Verification items for the finished model (mm, model axes). Give positions to 0.01 mm unless a question says otherwise; leave off trailing zeros. Order: outer loops, then holes, each group sorted by start corner. A loop starts at its lowest first (then second) coordinate and runs counter-clockwise, first axis right, second up.
from build123d import *
from OCP.BRepFilletAPI import BRepFilletAPI_MakeChamfer

# Parameters (mm, degrees)
SKETCH1_W           = 3.53
SKETCH1_H           = 9.2
BOSS_EXTRUDE1_DEPTH = 4
BOSS_EXTRUDE2_DEPTH = 4
CHAMFER1_SIZE       = 1.5
CHAMFER1_SIZE2      = 0.5
CHAMFER2_SIZE       = 0.5
CHAMFER2_SIZE2      = 1.5


with BuildPart() as part:
    # Sketch1 → Boss-Extrude1 (new body)
    with BuildSketch(Plane.XY):
        Polygon((52.4925, 30), (52.4925, -30), (-54.2075, -30), (-54.2075, 14), (-68.2075, 14), (-68.2075, 30), align=None)
        with BuildLine():
            Line((-31.510630119, 17.647843267), (22.89855475, 17.647843267))
            ThreePointArc((22.89855475, 17.647843267), (-4.306037684, -22.627990687), (-31.510630119, 17.647843267))
        make_face(mode=Mode.SUBTRACT)
        with Locations((-39.0075, 21.35)):
            Rectangle(SKETCH1_W, SKETCH1_H, mode=Mode.SUBTRACT)
        with Locations((45.7925, 20.65)):
            Rectangle(SKETCH1_W, SKETCH1_H, mode=Mode.SUBTRACT)
        with Locations((45.8, -20.65)):
            Rectangle(SKETCH1_W, SKETCH1_H, mode=Mode.SUBTRACT)
        with Locations((-64.9075, 21.35)):
            Rectangle(SKETCH1_W, SKETCH1_H, mode=Mode.SUBTRACT)
    extrude(amount=BOSS_EXTRUDE1_DEPTH)

    # Sketch2 → Boss-Extrude2 (add)
    with BuildSketch(Plane.XY):
        Polygon((-68.2075, 30), (52.4925, 30), (52.4925, 55), (37.4925, 55), (23.350364376, 40.857864376), (-39.065364376, 40.857864376), (-53.2075, 55), (-68.2075, 55), align=None)
    extrude(amount=BOSS_EXTRUDE2_DEPTH)

    # Chamfer1: one chamfer whose edges measure the first distance from different faces: ONE call of the kernel's chamfer builder (chamfer() names one face for all edges)
    chamfer1_edges_1 = [part.edges().sort_by_distance(p)[0] for p in [
        (-40.7725, 21.35, 0),
    ]]
    chamfer1_side_1 = [part.faces().sort_by_distance(p)[0] for p in [
        (-40.7725, 21.35, 2),
    ]]
    chamfer1_edges_2 = [part.edges().sort_by_distance(p)[0] for p in [
        (-39.0075, 16.75, 0),
    ]]
    chamfer1_side_2 = [part.faces().sort_by_distance(p)[0] for p in [
        (-39.0075, 16.75, 2),
    ]]
    chamfer1_edges_3 = [part.edges().sort_by_distance(p)[0] for p in [
        (-37.2425, 21.35, 0),
    ]]
    chamfer1_side_3 = [part.faces().sort_by_distance(p)[0] for p in [
        (-37.2425, 21.35, 2),
    ]]
    chamfer1_edges_4 = [part.edges().sort_by_distance(p)[0] for p in [
        (-39.0075, 25.95, 0),
    ]]
    chamfer1_side_4 = [part.faces().sort_by_distance(p)[0] for p in [
        (-39.0075, 25.95, 2),
    ]]
    chamfer1_edges_5 = [part.edges().sort_by_distance(p)[0] for p in [
        (-66.6725, 21.35, 0),
    ]]
    chamfer1_side_5 = [part.faces().sort_by_distance(p)[0] for p in [
        (-66.6725, 21.35, 2),
    ]]
    chamfer1_edges_6 = [part.edges().sort_by_distance(p)[0] for p in [
        (-64.9075, 16.75, 0),
    ]]
    chamfer1_side_6 = [part.faces().sort_by_distance(p)[0] for p in [
        (-64.9075, 16.75, 2),
    ]]
    chamfer1_edges_7 = [part.edges().sort_by_distance(p)[0] for p in [
        (-63.1425, 21.35, 0),
    ]]
    chamfer1_side_7 = [part.faces().sort_by_distance(p)[0] for p in [
        (-63.1425, 21.35, 2),
    ]]
    chamfer1_edges_8 = [part.edges().sort_by_distance(p)[0] for p in [
        (-64.9075, 25.95, 0),
    ]]
    chamfer1_side_8 = [part.faces().sort_by_distance(p)[0] for p in [
        (-64.9075, 25.95, 2),
    ]]
    chamfer1_edges_9 = [part.edges().sort_by_distance(p)[0] for p in [
        (44.0275, 20.65, 0),
    ]]
    chamfer1_side_9 = [part.faces().sort_by_distance(p)[0] for p in [
        (44.0275, 20.65, 2),
    ]]
    chamfer1_edges_10 = [part.edges().sort_by_distance(p)[0] for p in [
        (45.7925, 16.05, 0),
    ]]
    chamfer1_side_10 = [part.faces().sort_by_distance(p)[0] for p in [
        (45.7925, 16.05, 2),
    ]]
    chamfer1_edges_11 = [part.edges().sort_by_distance(p)[0] for p in [
        (47.5575, 20.65, 0),
    ]]
    chamfer1_side_11 = [part.faces().sort_by_distance(p)[0] for p in [
        (47.5575, 20.65, 2),
    ]]
    chamfer1_edges_12 = [part.edges().sort_by_distance(p)[0] for p in [
        (45.7925, 25.25, 0),
    ]]
    chamfer1_side_12 = [part.faces().sort_by_distance(p)[0] for p in [
        (45.7925, 25.25, 2),
    ]]
    chamfer1_edges_13 = [part.edges().sort_by_distance(p)[0] for p in [
        (47.565, -20.65, 0),
    ]]
    chamfer1_side_13 = [part.faces().sort_by_distance(p)[0] for p in [
        (47.565, -20.65, 2),
    ]]
    chamfer1_edges_14 = [part.edges().sort_by_distance(p)[0] for p in [
        (45.8, -16.05, 0),
    ]]
    chamfer1_side_14 = [part.faces().sort_by_distance(p)[0] for p in [
        (45.8, -16.05, 2),
    ]]
    chamfer1_edges_15 = [part.edges().sort_by_distance(p)[0] for p in [
        (44.035, -20.65, 0),
    ]]
    chamfer1_side_15 = [part.faces().sort_by_distance(p)[0] for p in [
        (44.035, -20.65, 2),
    ]]
    chamfer1_edges_16 = [part.edges().sort_by_distance(p)[0] for p in [
        (45.8, -25.25, 0),
    ]]
    chamfer1_side_16 = [part.faces().sort_by_distance(p)[0] for p in [
        (45.8, -25.25, 2),
    ]]
    chamfer1 = BRepFilletAPI_MakeChamfer(part.part.solid().wrapped)
    for e in chamfer1_edges_1:
        chamfer1.Add(CHAMFER1_SIZE, CHAMFER1_SIZE2, e.wrapped, chamfer1_side_1[0].wrapped)  # the first distance lies on this face
    for e in chamfer1_edges_2:
        chamfer1.Add(CHAMFER1_SIZE, CHAMFER1_SIZE2, e.wrapped, chamfer1_side_2[0].wrapped)  # the first distance lies on this face
    for e in chamfer1_edges_3:
        chamfer1.Add(CHAMFER1_SIZE, CHAMFER1_SIZE2, e.wrapped, chamfer1_side_3[0].wrapped)  # the first distance lies on this face
    for e in chamfer1_edges_4:
        chamfer1.Add(CHAMFER1_SIZE, CHAMFER1_SIZE2, e.wrapped, chamfer1_side_4[0].wrapped)  # the first distance lies on this face
    for e in chamfer1_edges_5:
        chamfer1.Add(CHAMFER1_SIZE, CHAMFER1_SIZE2, e.wrapped, chamfer1_side_5[0].wrapped)  # the first distance lies on this face
    for e in chamfer1_edges_6:
        chamfer1.Add(CHAMFER1_SIZE, CHAMFER1_SIZE2, e.wrapped, chamfer1_side_6[0].wrapped)  # the first distance lies on this face
    for e in chamfer1_edges_7:
        chamfer1.Add(CHAMFER1_SIZE, CHAMFER1_SIZE2, e.wrapped, chamfer1_side_7[0].wrapped)  # the first distance lies on this face
    for e in chamfer1_edges_8:
        chamfer1.Add(CHAMFER1_SIZE, CHAMFER1_SIZE2, e.wrapped, chamfer1_side_8[0].wrapped)  # the first distance lies on this face
    for e in chamfer1_edges_9:
        chamfer1.Add(CHAMFER1_SIZE, CHAMFER1_SIZE2, e.wrapped, chamfer1_side_9[0].wrapped)  # the first distance lies on this face
    for e in chamfer1_edges_10:
        chamfer1.Add(CHAMFER1_SIZE, CHAMFER1_SIZE2, e.wrapped, chamfer1_side_10[0].wrapped)  # the first distance lies on this face
    for e in chamfer1_edges_11:
        chamfer1.Add(CHAMFER1_SIZE, CHAMFER1_SIZE2, e.wrapped, chamfer1_side_11[0].wrapped)  # the first distance lies on this face
    for e in chamfer1_edges_12:
        chamfer1.Add(CHAMFER1_SIZE, CHAMFER1_SIZE2, e.wrapped, chamfer1_side_12[0].wrapped)  # the first distance lies on this face
    for e in chamfer1_edges_13:
        chamfer1.Add(CHAMFER1_SIZE, CHAMFER1_SIZE2, e.wrapped, chamfer1_side_13[0].wrapped)  # the first distance lies on this face
    for e in chamfer1_edges_14:
        chamfer1.Add(CHAMFER1_SIZE, CHAMFER1_SIZE2, e.wrapped, chamfer1_side_14[0].wrapped)  # the first distance lies on this face
    for e in chamfer1_edges_15:
        chamfer1.Add(CHAMFER1_SIZE, CHAMFER1_SIZE2, e.wrapped, chamfer1_side_15[0].wrapped)  # the first distance lies on this face
    for e in chamfer1_edges_16:
        chamfer1.Add(CHAMFER1_SIZE, CHAMFER1_SIZE2, e.wrapped, chamfer1_side_16[0].wrapped)  # the first distance lies on this face
    add(Compound.cast(chamfer1.Shape()), mode=Mode.REPLACE)

    # Chamfer2
    chamfer2_edges = [part.edges().sort_by_distance(p)[0] for p in [
        (-40.7725, 21.35, 4),
        (-39.0075, 16.75, 4),
        (-37.2425, 21.35, 4),
        (-39.0075, 25.95, 4),
        (-66.6725, 21.35, 4),
        (-64.9075, 16.75, 4),
        (-63.1425, 21.35, 4),
        (-64.9075, 25.95, 4),
        (44.0275, 20.65, 4),
        (45.7925, 16.05, 4),
        (47.5575, 20.65, 4),
        (45.7925, 25.25, 4),
        (47.565, -20.65, 4),
        (45.8, -16.05, 4),
        (44.035, -20.65, 4),
        (45.8, -25.25, 4),
    ]]
    chamfer2_side = [part.faces().sort_by_distance(p)[0] for p in [
        (-0.8575, -28.523738167, 4),
    ]]
    chamfer(chamfer2_edges, length=CHAMFER2_SIZE, length2=CHAMFER2_SIZE2, reference=chamfer2_side[0])


solid = part.part
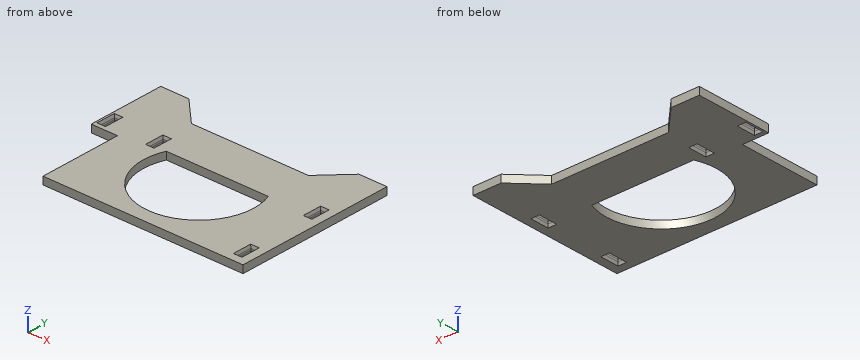
(1) Section check D-D, the plane z = 3.35. Enter the section's corners in (x, y).
Solved:
outline: (-68.21, 14) - (-54.21, 14) - (-54.21, -30) - (52.49, -30) - (52.49, 55) - (37.49, 55) - (23.35, 40.86) - (-39.07, 40.86) - (-53.21, 55) - (-68.21, 55) - close; hole (-66.96, 16.47) - (-62.86, 16.47) - (-62.86, 26.23) - (-66.96, 26.23) - close; hole (-41.06, 16.47) - (-36.96, 16.47) - (-36.96, 26.23) - (-41.06, 26.23) - close; hole (-31.51, 17.65) arc R29.33 ccw (long way) to (22.9, 17.65) - close; hole (43.74, 15.77) - (47.84, 15.77) - (47.84, 25.53) - (43.74, 25.53) - close; hole (43.75, -25.53) - (47.85, -25.53) - (47.85, -15.77) - (43.75, -15.77) - close
(2) Section check B-B, the plane y = -19. Enter the section's corners in (x, z) (1 decimal), then the cut area to 3 significant figures.
Solved:
outline: (-54.2, 0) - (-18.4, 0) - (-18.4, 4) - (-54.2, 4) - close; (9.8, 0) - (43.5, 0) - (44, 1.5) - (44, 2.5) - (43.5, 4) - (9.8, 4) - close; (47.6, 1.5) - (48.1, 0) - (52.5, 0) - (52.5, 4) - (48.1, 4) - (47.6, 2.5) - close
area: 298 mm2
(3) Scan lines: line 1 (Y direction, x = 46, z = 2); line 2 (X direction, y = -19, z = 1.15); line 3 (X direction, y = -19.5, z = 1.3). Record each from-to range of solid material in increasing order.
Solved:
line 1: y = -30 to -25.25, -16.05 to 16.05, 25.25 to 55
line 2: x = -54.21 to -18.43, 9.82 to 43.92, 47.68 to 52.49
line 3: x = -54.21 to -17.48, 8.87 to 43.97, 47.63 to 52.49
(4) Section check C-C, the plane y = -1. Enter the section's corners in (x, z), then the cut area to 3 significant figures.
Solved:
outline: (-54.21, 0) - (-32.6, 0) - (-32.6, 4) - (-54.21, 4) - close; (23.99, 0) - (52.49, 0) - (52.49, 4) - (23.99, 4) - close
area: 200 mm2
(5) Go/stop test with flat-tipped pins: pin 1 (0.8 mm diameter, centred on x = -39.5, z = 2, fed in from +Y); pin 2 (1.5 mm diameter, centred on y = 9, z = 2, fed in from -X); pin 3 (0.8 mm diameter, centred on x = -65, z = 2, fed in from -Y). Record where each tip stops, or that it passes through.
Solved:
pin 1: stops at y = 41.69
pin 2: stops at x = -54.21
pin 3: stops at y = 14
(6) Section check A-A, the plane x = -16. Enter the section's corners in (y, z).
Solved:
outline: (-30, 0) - (-20.2, 0) - (-20.2, 4) - (-30, 4) - close; (17.65, 0) - (40.86, 0) - (40.86, 4) - (17.65, 4) - close
